Could you check a few things on this model? Use its own coordinates, in mm. A direction names the side the tool comes from. Round coordinates to 2 decimals unless told otherwise and drop trailing zeros. Order: outer loops, then holes, each group sorted by start corner. A loop starts at its lowest first (then second) coordinate and runs counter-clockwise, first axis right, second up. Notation, with made-up numbers: (-24, 3) - (35, 3) arc R20 ccw to (35, 32) - close; hole circle Ø4 at (49.25, -38). An arc over 180 degrees is marked (long way). Return JSON: item names as keys, results as strings. Group by question number.
from build123d import *

# Parameters (mm, degrees)
BOSS_EXTRUDE2_DEPTH = 15.95
SKETCH2_R           = 2.445
BOSS_EXTRUDE3_DEPTH = 1.81
SKETCH3_W           = 8.01
SKETCH3_H           = 7.975
BOSS_EXTRUDE4_DEPTH = 6.6
SKETCH4_R           = 2.455
SKETCH4_R_2         = 1.525
BOSS_EXTRUDE5_DEPTH = 1.74


with BuildPart() as part:
    # Sketch1 → Boss-Extrude2 (new body)
    with BuildSketch(Plane.XY):
        Polygon((-7.965, 9.74), (7.965, 9.74), (7.965, 0), (15.975, 0), (15.975, -3.4), (-15.975, -3.4), (-15.975, 0), (-7.965, 0), align=None)
    extrude(amount=-BOSS_EXTRUDE2_DEPTH)

    # Sketch2 → Boss-Extrude3 (add)
    with BuildSketch(Plane(origin=(0, 9.74, 0), x_dir=(1, 0, 0), z_dir=(0, 1, 0))):
        with Locations(Location((-3.985, 11.97, 0), (0, 0, 270))):
            Circle(SKETCH2_R)
        with Locations(Location((3.975, 11.97, 0), (0, 0, 270))):
            Circle(SKETCH2_R)
        with Locations(Location((3.975, 4.01, 0), (0, 0, 270))):
            Circle(SKETCH2_R)
        with Locations(Location((-3.985, 4.01, 0), (0, 0, 270))):
            Circle(SKETCH2_R)
    extrude(amount=BOSS_EXTRUDE3_DEPTH)

    # Sketch3 → Boss-Extrude4 (add)
    with BuildSketch(Plane(origin=(0, 0, 0), x_dir=(1, 0, 0), z_dir=(0, 1, 0))):
        with Locations((-11.97, 11.9625)):
            Rectangle(SKETCH3_W, SKETCH3_H)
        with Locations((11.97, 11.9625)):
            Rectangle(SKETCH3_W, SKETCH3_H)
    extrude(amount=BOSS_EXTRUDE4_DEPTH)

    # Sketch4 → Boss-Extrude5 (add)
    # profile 1 of 2: a face of its own
    with BuildSketch(Plane(origin=(0, 6.6, 0), x_dir=(1, 0, 0), z_dir=(0, 1, 0))):
        with Locations(Location((11.97, 11.96, 0), (0, 0, 270))):
            Circle(SKETCH4_R)
        with Locations(Location((11.97, 11.96, 0), (0, 0, 270))):
            Circle(SKETCH4_R_2, mode=Mode.SUBTRACT)
    # profile 2 of 2: a face of its own
    with BuildSketch(Plane(origin=(0, 6.6, 0), x_dir=(1, 0, 0), z_dir=(0, 1, 0))):
        with Locations(Location((-11.97, 11.96, 0), (0, 0, 90))):
            Circle(SKETCH4_R)
        with Locations(Location((-11.97, 11.96, 0), (0, 0, 90))):
            Circle(SKETCH4_R_2, mode=Mode.SUBTRACT)
    extrude(amount=BOSS_EXTRUDE5_DEPTH)


solid = part.part
1) For faces 1 (the flat face through (0, 9.74, -8)), 2 (the flat face through (-12, 8.34, -14)), 3 (the flat face through (12, 0, -4)), which set-ups out of +Z, -Z, +X, -X, +Y, -Y let a thin tool reach every point of the face, with its end or its side?
2) I want a section at A-A, the plane z = -4.01. List the corners of the cut face in (x, y) for me (3 decimals).
3) I want a section at D-D, the plane z = -1.25. List the corners of the cut face in (x, y) for me (3 decimals).
4) I want a section at C-C, the plane y = 4.25. List the corners of the cut face in (x, z) for me (3 decimals).
5) Will these pins go through, and if not, where does the flat tip stop? pin 1 (6.5 mm diameter, centred on x = 10.5, z = -10.5, fed in from +Y); pin 2 (2.5 mm diameter, centred on x = -11.97, z = -11.96, fed in from +Y); pin 3 (4 mm diameter, centred on x = 11.97, z = -11.96, fed in from +Y).
6) I want a section at B-B, the plane x = 11.97. List the corners of the cut face in (y, z) for me (3 decimals).
7) If I drill on line 1 along X through (y, z) = (7, -11.96) (3 decimals); line 2 along Z through (x, y) = (-11.97, 7.15) (3 decimals); line 3 along X through (y, z) = (5.25, -1.25) (3 decimals), over which ranges is the centre line in solid material (lowest first)? Write a range as from..to.
Outcome:
{
 "1": {"face 1": "+Y", "face 2": "+Z, -Z, -X, +Y", "face 3": "+Z, +X, +Y"},
 "2": {"outline": "(-15.975, -3.4) - (15.975, -3.4) - (15.975, 0) - (7.965, 0) - (7.965, 9.74) - (6.42, 9.74) - (6.42, 11.55) - (1.53, 11.55) - (1.53, 9.74) - (-1.54, 9.74) - (-1.54, 11.55) - (-6.43, 11.55) - (-6.43, 9.74) - (-7.965, 9.74) - (-7.965, 0) - (-15.975, 0) - close"},
 "3": {"outline": "(-15.975, -3.4) - (15.975, -3.4) - (15.975, 0) - (7.965, 0) - (7.965, 9.74) - (-7.965, 9.74) - (-7.965, 0) - (-15.975, 0) - close"},
 "4": {"outline": "(-15.975, -15.95) - (15.975, -15.95) - (15.975, -7.975) - (7.965, -7.975) - (7.965, 0) - (-7.965, 0) - (-7.965, -7.975) - (-15.975, -7.975) - close"},
 "5": {"pin 1": "y = 9.74", "pin 2": "y = 6.6", "pin 3": "y = 8.34"},
 "6": {"outline": "(-3.4, -15.95) - (6.6, -15.95) - (6.6, -14.415) - (8.34, -14.415) - (8.34, -13.485) - (6.6, -13.485) - (6.6, -10.435) - (8.34, -10.435) - (8.34, -9.505) - (6.6, -9.505) - (6.6, -7.975) - (0, -7.975) - (0, 0) - (-3.4, 0) - close"},
 "7": {"line 1": "-14.425..-13.495, -10.445..-9.515, -7.965..7.965, 9.515..10.445, 13.495..14.425", "line 2": "-14.415..-13.485, -10.435..-9.505", "line 3": "-7.965..7.965"}
}
